Check sheet for the modelled part. Datum: model origin and axes. Units: mm. Give positions to 0.01 mm unless a question says otherwise; leave off trailing zeros. Loops run counter-clockwise (first coordinate to the right, second up) from the corner with the lowest first, then second, coordinate; pieces in that order, holes last. Notation, with made-up numbers: M 58.25,11.5 L 72.25,11.5 A22 cw 72.25,37.5 Z; hole C 82.5,57.5 d3. An arc over 180 degrees is marked long. One line per question, with ' | ' between items. Start each with the question number.
from build123d import *

# Parameters (mm, degrees)
EXTRUDE_THIN1_DEPTH = 2300
SKETCH2_R           = 3.25
CUT_EXTRUDE1_DEPTH  = 10
LPATTERN1_COUNT     = 3
LPATTERN1_PITCH     = 766


with BuildPart() as part:
    # Sketch1 → Extrude-Thin1 (new body)
    with BuildSketch(Plane.XY):
        with BuildLine():
            Line((16.84, 2), (16.84, -23))
            ThreePointArc((16.84, -23), (15.961320344, -25.121320344), (13.84, -26))
            Line((13.84, -26), (-17.16, -26))
            ThreePointArc((-17.16, -26), (-19.281320344, -25.121320344), (-20.16, -23))
            Line((-20.16, -23), (-20.16, 2))
            Line((-20.16, 2), (-18.66, 2))
            Line((-18.66, 2), (-18.66, -23))
            ThreePointArc((-18.66, -23), (-18.220660172, -24.060660172), (-17.16, -24.5))
            Line((-17.16, -24.5), (13.84, -24.5))
            ThreePointArc((13.84, -24.5), (14.900660172, -24.060660172), (15.34, -23))
            Line((15.34, -23), (15.34, 2))
            Line((15.34, 2), (16.84, 2))
        make_face()
    extrude(amount=EXTRUDE_THIN1_DEPTH)

    # Sketch2 → Cut-Extrude1 (cut)
    with BuildSketch(Plane(origin=(0, -24.5, 0), x_dir=(1, 0, 0), z_dir=(0, 1, 0))):
        with Locations(Location((0, -383, 0), (0, 0, 270))):
            Circle(SKETCH2_R)
    cut_extrude1 = extrude(amount=-CUT_EXTRUDE1_DEPTH, mode=Mode.SUBTRACT)

    # LPattern1: Cut-Extrude1 ×3
    with Locations(*[(0, 0, i * LPATTERN1_PITCH) for i in range(1, LPATTERN1_COUNT)]):
        add(cut_extrude1, mode=Mode.SUBTRACT)


solid = part.part
Q1. Depth check by flat-ended pin: P1, Ø8.5, axis at x = 0, z = 1149, coming from the -Y side; P2, Ø9.5, axis at x = 0, z = 1638, coming from the +Y side; P3, Ø1.5, axis at x = 13, y = -5.5, coming from the -Z side. Enter the tip coordinate at first touch or a pass-through.
Q2. Material ranges on probe 1 along X at (y, z) = (-25.3, 1915); probe 2 along X at (y, z) = (-25.6, 383); probe 3 along Y at (x, z) = (-11, 244), recorded low to high. Write a range as from..to.
Q3. Cross-section at B-B (x = -9). Record the cut outline in (y, z).
Q4. Cross-section at A-A (z = 175). Record the cut outline in (x, y), and give its area (3 significant figures).
Solved:
1) P1: stops at y = -26 | P2: stops at y = -24.5 | P3: passes through
2) probe 1: x = -19.09..-3.25, 3.25..15.77 | probe 2: x = -18.66..-3.25, 3.25..15.34 | probe 3: y = -26..-24.5
3) outline: M -26,0 L -24.5,0 L -24.5,2300 L -26,2300 Z
4) outline: M -20.16,-23 A3 ccw -17.16,-26 L 13.84,-26 A3 ccw 16.84,-23 L 16.84,2 L 15.34,2 L 15.34,-23 A1.5 cw 13.84,-24.5 L -17.16,-24.5 A1.5 cw -18.66,-23 L -18.66,2 L -20.16,2 Z | area: 132 mm²
